Part model, mm, in its own coordinate system. A direction names the side the tool comes from. Coordinates: 2 decimals unless noted, no trailing zeros. Write each loop counter-clockwise with the first axis right and the second up, starting at its lowest first coordinate (ties: lowest second). Pieces come first, ordered by that corner, then holes. Notation, with made-up numbers: (76.25, -1.5) - (115.25, -1.5) arc R22 cw to (115.25, 7.5) - close; hole circle Ø11 at (37.25, 88). An arc over 180 degrees is marked (long way). Write each question's results on one line, items separated by ' | '.
Autodesk Inventor part; units mm, degrees
ref_plane "YZ Plane" through (0, 0, 0) normal (1, 0, 0) x (0, 1, 0)
ref_plane "XZ Plane" through (0, 0, 0) normal (0, 1, 0) x (-1, 0, 0)
ref_plane "XY Plane" through (0, 0, 0) normal (0, 0, 1) x (1, 0, 0)
sketch "Sketch1" plane through (0, 0, 0) normal (0, 0, 1) x (1, 0, 0)
  line L0 (0, 0) -> (0, 14.351)
  line L1 (0, 0) -> (14.351, 0) construction
  line L2 (0, 14.351) -> (16.51, 14.351)
  line L3 (16.51, 14.351) -> (16.51, 27.051)
  line L4 (16.51, 27.051) -> (34.29, 27.051)
  line L5 (34.29, 27.051) -> (34.29, 12.7)
  line L6 (34.29, 12.7) -> (12.7, 12.7)
  line L7 (12.7, 12.7) -> (12.7, 0)
  line L8 (0, 0) -> (12.7, 0)
  dimension "d0" = 14.351
  dimension "d2" = 16.51
  dimension "d6" = 17.78
  dimension "d9" = 21.59
  dimension "d47" = 14.351
  dimension "d49" = 12.7
extrude "Extrusion1" add sketch "Sketch1" along normal blind 127
sketch "Sketch3" plane through (16.51, 27.051, 0) normal (0, 1, 0) x (1, 0, 0)
  line L0 (0, -127) -> (-16.51, -127)
  line L1 (-16.51, 0) -> (0, 0)
  line L2 (-16.51, 0) -> (-16.51, -127)
  point P0 (-10.16, -12.7)
  point P1 (-10.16, -114.3)
  dimension "d25" = 12.7
  dimension "d26" = 12.7
  dimension "d27" = 6.35
  dimension "d28" = 6.35
hole "Hole2" at (6.35, 27.051, 12.7) at (6.35, 27.051, 114.3) direction (0, -1, 0) diameter 9.525 end through all
sketch "Sketch4" plane through (16.51, 27.051, 0) normal (0, 1, 0) x (1, 0, 0)
  line L0 (17.78, 0) -> (17.78, -127)
  line L1 (17.78, -127) -> (0, -127)
  line L2 (0, 0) -> (17.78, 0)
  line L3 (0, 0) -> (0, -127)
  point P0 (-16.51, 0)
  point P1 (8.89, -12.7)
  point P2 (8.89, -114.3)
  dimension "d36" = 8.89
  dimension "d37" = 12.7
  dimension "d38" = 12.7
  dimension "d48" = 17.78
hole "Hole3" at (25.4, 27.051, 12.7) at (25.4, 27.051, 114.3) direction (0, -1, 0) diameter 15.875 end through all
sketch "Sketch5" plane through (16.51, 27.051, 0) normal (0, 1, 0) x (1, 0, 0)
  line L0 (3.81, -101.6) -> (13.335, -101.6)
  line L1 (13.335, -101.6) -> (13.335, -25.4)
  line L2 (13.335, -25.4) -> (3.81, -25.4)
  line L3 (3.81, -25.4) -> (3.81, -101.6)
  line L4 (17.78, -127) -> (0, -127)
  line L5 (17.78, 0) -> (17.78, -127)
  line L6 (0, 0) -> (17.78, 0)
  point P0 (-16.51, 0)
  dimension "d50" = 25.4
  dimension "d51" = 4.445
  dimension "d52" = 25.4
  dimension "d53" = 9.525
extrude "Extrusion2" cut sketch "Sketch5" against normal blind 25.4
sketch "Sketch6" plane through (0, 0, 0) normal (0, -1, 0) x (1, 0, 0)
  line L0 (3.81, 25.4) -> (8.89, 25.4)
  line L1 (8.89, 25.4) -> (8.89, 101.6)
  line L2 (8.89, 101.6) -> (3.81, 101.6)
  line L3 (3.81, 101.6) -> (3.81, 25.4)
  line L4 (20.32, 101.6) -> (29.845, 101.6)
  line L5 (29.845, 25.4) -> (20.32, 25.4)
  line L6 (0, 0) -> (0, 127)
  line L7 (12.7, 0) -> (12.7, 127)
  dimension "d57" = 3.81
  dimension "d58" = 3.81
extrude "Extrusion3" cut sketch "Sketch6" against normal blind 25.4
fillet "Fillet1" radius 1.905 8 edges at (20.32, 19.8755, 25.4) (29.845, 19.8755, 25.4) (20.32, 19.8755, 101.6) (29.845, 19.8755, 101.6) (3.81, 7.1755, 101.6) (8.89, 7.1755, 101.6) (8.89, 7.1755, 25.4) (3.81, 7.1755, 25.4)
chamfer "Chamfer1" distance 5.08 angle 45 2 edges at (16.51, 14.351, 63.5) (12.7, 12.7, 63.5)
sketch "Sketch7" plane through (0, 14.351, 127) normal (0, 1, 0) x (1, 0, 0)
  circle A0 centre (6.35, 114.3) radius 4.7625
  circle A1 centre (6.35, 114.3) radius 8.001
  circle A2 centre (6.35, 12.7) radius 4.7625
  circle A3 centre (6.35, 12.7) radius 8.001
  point P0 (0, 127)
  dimension "d65" = 16.002
  dimension "d66" = 16.002
extrude "Extrusion4" cut sketch "Sketch7" against normal blind 3.81
sketch "Sketch8" plane through (0, 14.351, 0) normal (0, 1, 0) x (1, 0, 0)
  arc A0 (0, -17.5676) -> (11.43, -18.8814) centre (6.35, -12.7) ccw
  circle A1 centre (6.35, -12.7) radius 8.001
  arc A2 (11.43, -108.1186) -> (0, -109.4324) centre (6.35, -114.3) ccw
  circle A3 centre (6.35, -114.3) radius 8.001
  point P0 (0, 0)
extrude "Extrusion5" cut sketch "Sketch8" along normal blind 3.81
chamfer "Chamfer2" distance 2.54 angle 45 1 edges at (34.29, 12.7, 63.5)
equation "\"d0\" = d47"
equation "\"d58\" = d57"
properties part number "Block_3-8" material "Aluminum 6061"
(1) Wall check: line 1 (Z direction, x = 6.35, y = 7.5); line 2 (Z direction, x = 25.4, y = 24); line 3 (X direction, y = 20.75, z = 12.7). Give the ranges that are in metal, low to high. Write a range as from..to.
Return value:
line 1: z = 0..7.94, 17.46..25.4, 101.6..109.54, 119.06..127 | line 2: z = 0..4.76, 20.64..25.4, 101.6..106.36, 122.24..127 | line 3: x = 16.51..17.46, 33.34..34.29
(2) Saw through at D-D on z = 12.7. Write the cut outline in (x, y).
Return value:
outline: (0, 0) - (1.59, 0) - (1.59, 10.54) - (0, 10.54) - close; (11.11, 0) - (12.7, 0) - (12.7, 7.62) - (17.46, 12.38) - (17.46, 27.05) - (16.51, 27.05) - (16.51, 19.43) - (14.35, 17.27) - (14.35, 10.54) - (11.11, 10.54) - close; (33.34, 14.29) - (34.29, 15.24) - (34.29, 27.05) - (33.34, 27.05) - close
(3) Saw through at A-A on x = 25.4. Write the cut outline in (y, z), then the cut area to 3 significant figures.
Return value:
outline: (12.7, 0) - (27.05, 0) - (27.05, 4.76) - (12.7, 4.76) - close; (12.7, 20.64) - (27.05, 20.64) - (27.05, 25.4) - (12.7, 25.4) - close; (12.7, 101.6) - (27.05, 101.6) - (27.05, 106.36) - (12.7, 106.36) - close; (12.7, 122.24) - (27.05, 122.24) - (27.05, 127) - (12.7, 127) - close | area: 273 mm^2
(4) 3-axis set-ups, long thin cutter, end or side, ignore diameter. For faces 1 (the flat face through (20, 12.7, 74)), 2 (the flat face through (3, 14.351, 63)), 3 (the flat face through (20.32, 20, 63)), 4 (the flat face through (9.1, 0, 62.6)): which of +Z, -Z, +X, -X, +Y, -Y reach the whole face in a straight line?
Return value:
face 1: +Z, -Z, +X, -Y | face 2: +Z, -Z, -X, +Y | face 3: +Y, -Y | face 4: +Z, -Z, +X, -X, -Y
(5) Saw through at B-B on z = 72. Write the cut outline in (x, y) (3 decimals).
Return value:
outline: (0, 0) - (3.81, 0) - (3.81, 14.351) - (0, 14.351) - close; (8.89, 0) - (12.7, 0) - (12.7, 7.62) - (17.78, 12.7) - (20.32, 12.7) - (20.32, 27.051) - (16.51, 27.051) - (16.51, 19.431) - (11.43, 14.351) - (8.89, 14.351) - close; (29.845, 12.7) - (31.75, 12.7) - (34.29, 15.24) - (34.29, 27.051) - (29.845, 27.051) - close
(6) Saw through at C-C on x = 10. Write the cut outline in (y, z).
Return value:
outline: (0, 0) - (14.35, 0) - (14.35, 5.58) - (10.54, 5.58) - (10.54, 9.64) - (0, 9.64) - close; (0, 15.76) - (10.54, 15.76) - (10.54, 19.82) - (14.35, 19.82) - (14.35, 107.18) - (10.54, 107.18) - (10.54, 111.24) - (0, 111.24) - close; (0, 117.36) - (10.54, 117.36) - (10.54, 121.42) - (14.35, 121.42) - (14.35, 127) - (0, 127) - close
(7) Two-plate mould, pull along X, no slides. Class faces 5 (the flat face through (8.89, 7, 63)), 6 (the flat face through (29.845, 20, 64)), 7 (the flat face through (13.934, 16.855, 62.611)), 8 (the flat face through (12.7, 4, 63)): released by +X, released by -X, zero draft, split by the parting line, or undercut.
Return value:
face 5: undercut | face 6: undercut | face 7: released by -X | face 8: released by +X
(8) Flat gauge pins, fed straight in: P1, Ø1.5, axis at x = 19, y = 19.5, coming from the -Z side; P2, Ø6.5, axis at x = 3, z = 123.5, coming from the +Y side; P3, Ø4, axis at y = 16.5, z = 107.5, coming from the -X side; P4, Ø11.5, axis at y = 4.5, z = 71, coming from the +X side. Where does each tip first touch, or does it go through?
Return value:
P1: stops at z = 0 | P2: stops at y = 14.35 | P3: stops at x = 11.58 | P4: stops at x = 15.33
